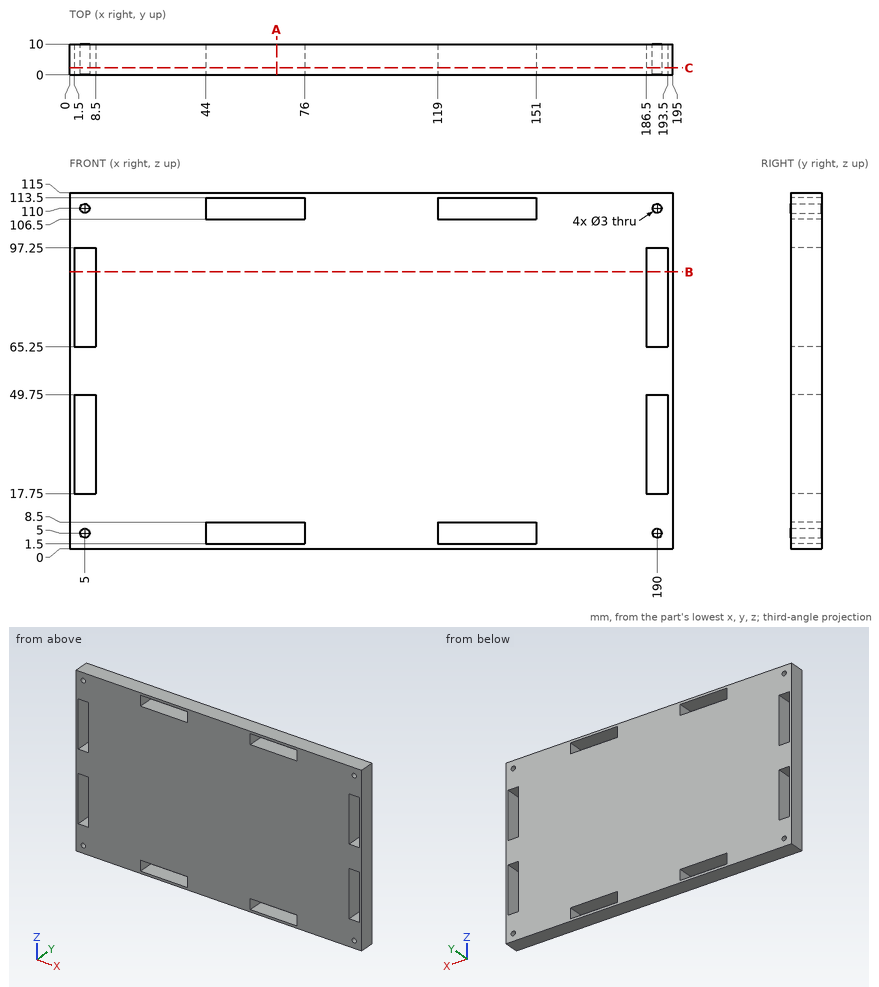
Here's the drawing with two shaded views (mm, measured from the low corner). I have some questions. Give positions to 0.01 mm unless a question says otherwise; leave off trailing zeros. Loops run counter-clockwise (first coordinate to the right, second up) from the corner with the lowest first, then second, coordinate; pieces in that order, holes last. Notation, with made-up numbers: (49, 2) - (85, 2) arc R18 cw to (85, 31) - close; hole circle Ø4 at (79, 65). An arc over 180 degrees is marked (long way). Answer in a Markdown table with one row per item. Add a question column.
Q1. Please list where these lines run through material, in increasing order: L1, parallel to X at y = 2.5, z = 5; L2, parallel to Z at x = 51, y = 7.5; L3, parallel to Z at x = 190, y = 2. Write a range as from..to.
Q2. If we section it at B-B (z = 89.5): List the corners of the cut face in (x, y) for me.
Q3. If we section it at A-A (x = 67): List the corners of the cut face in (y, z) for me, plus the area to 3 significant figures.
Q4. If we section it at C-C (y = 2.25): State how many separate pieces and enclosed holes the cut face has, plus the area to 3 significant figures.
Q5. For pin 1 (6 mm diameter, centred on y = 2, z = 54.5, fed in from -X), with a flat end and sliding along its axis, tell me the tip position at first contact or that it passes through.
The answers:
| question | item | result |
|---|---|---|
| 1 | L1 | x = 0..3.5, 6.5..44, 76..119, 151..188.5, 191.5..195 |
| 1 | L2 | z = 0..1.5, 8.5..106.5, 113.5..115 |
| 1 | L3 | z = 0..3.5, 6.5..17.75, 49.75..65.25, 97.25..108.5, 111.5..115 |
| 2 | outline | (0, 0) - (1.5, 0) - (1.5, 10) - (0, 10) - close; (8.5, 0) - (186.5, 0) - (186.5, 10) - (8.5, 10) - close; (193.5, 0) - (195, 0) - (195, 10) - (193.5, 10) - close |
| 3 | outline | (0, 0) - (10, 0) - (10, 1.5) - (0, 1.5) - close; (0, 8.5) - (10, 8.5) - (10, 106.5) - (0, 106.5) - close; (0, 113.5) - (10, 113.5) - (10, 115) - (0, 115) - close |
| 3 | area | 1,010 mm^2 |
| 4 | separate pieces | 1 |
| 4 | enclosed holes | 12 |
| 4 | area | 20,600 mm^2 |
| 5 | pin 1 | stops at x = 0 |
